Here's the drawing with two shaded views (mm, measured from the low corner). I have some questions. Give positions to 0.01 mm unless a question says otherwise; leave off trailing zeros. Write each loop counter-clockwise with the first axis right and the second up, starting at its lowest first coordinate (ties: lowest second). Pieces come first, ordered by that corner, then holes. Notation, with made-up numbers: (50, 80.5) - (87, 80.5) arc R21 ccw to (87, 103.5) - close; hole circle Ø7 at (-31.75, 70.25). An arc over 180 degrees is marked (long way). Use one line per item in the form item = value.
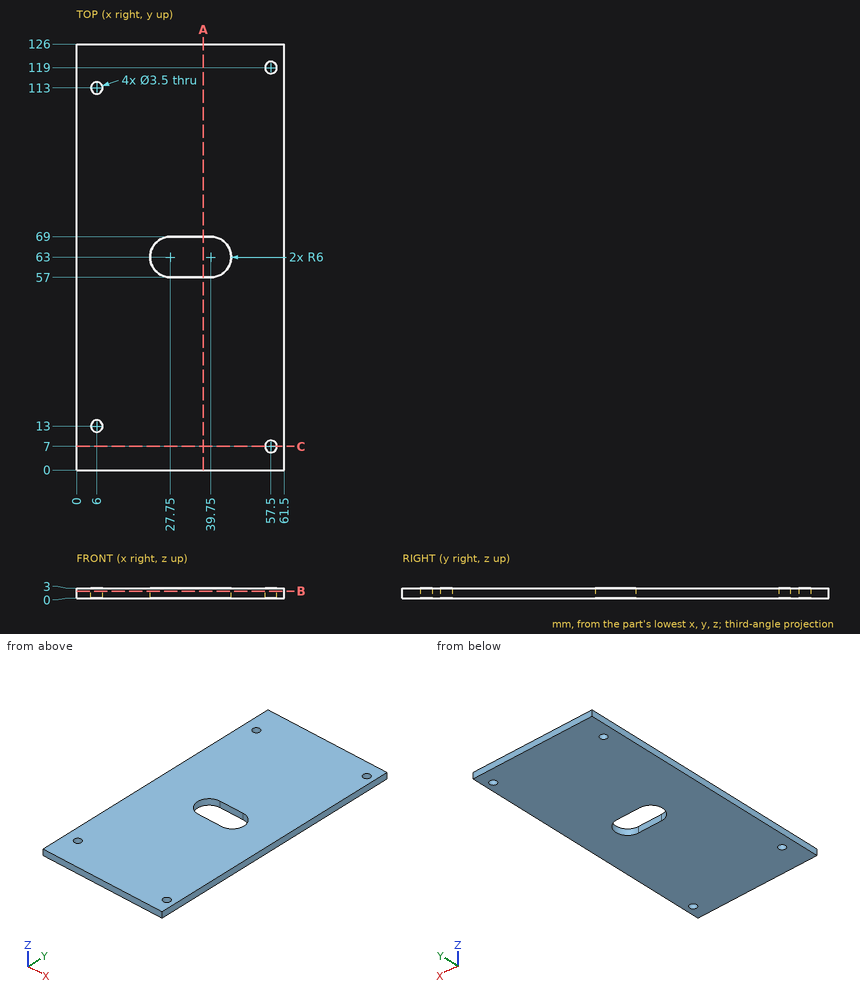
1. For pin 1 (2 mm diameter, centred on x = 57.5, y = 7, fed in from -Z), with a flat end and sliding along its axis, tell me the tip position at first contact or that it passes through.
Response values:
pin_1 = through
2. Imagine slicing it at B-B, the plane z = 2.1. List the corners of the cut face in (x, y) for me.
Response values:
outline = (0, 0) - (61.5, 0) - (61.5, 126) - (0, 126) - close; hole circle Ø3.5 at (6, 13); hole circle Ø3.5 at (6, 113); hole (27.75, 57) - (39.75, 57) arc R6 ccw to (39.75, 69) - (27.75, 69) arc R6 ccw to start; hole circle Ø3.5 at (57.5, 7); hole circle Ø3.5 at (57.5, 119)
3. Imagine slicing it at A-A, the plane x = 37.5. List the corners of the cut face in (y, z) for me, and give its area (3 significant figures).
Response values:
outline = (0, 0) - (57, 0) - (57, 3) - (0, 3) - close; (69, 0) - (126, 0) - (126, 3) - (69, 3) - close
area = 342 mm²
4. If I drill on line 1 (Y direction, x = 6, z = 2); line 2 (Y direction, x = 57.5, z = 1.4); line 3 (X direction, y = 119, z = 1.8), over which ranges is the centre line in solid material (lowest first)? Write a range as from..to.
Response values:
line_1 = 0..11.25, 14.75..111.25, 114.75..126
line_2 = 0..5.25, 8.75..117.25, 120.75..126
line_3 = 0..55.75, 59.25..61.5
5. Imagine slicing it at C-C, the plane y = 7. List the corners of the cut face in (x, z) for me.
Response values:
outline = (0, 0) - (55.75, 0) - (55.75, 3) - (0, 3) - close; (59.25, 0) - (61.5, 0) - (61.5, 3) - (59.25, 3) - close
